Verification items for this drawing (mm, ordinates from the low corner). A direction names the side the tool comes from. Coordinates: 2 decimals unless noted, no trailing zeros. Order: outer loops, then holes, each group sorted by start corner. A loop starts at its lowest first (then second) coordinate and runs counter-clockwise, first axis right, second up. Notation, with made-up numbers: M -7,24 L 6,24 A25 ccw 6,51 Z; hole C 61.5,8.25 d2. An arc over 180 degrees is marked long. One line per item, written item: value. Start each with the question number.
1) Thickness scan on L1, parallel to X at y = 4.05, z = 8; L2, parallel to X at y = 5.75, z = 39; L3, parallel to Z at x = 12, y = 4.25 (1 decimal). Record the ranges inside material, lowest first. Write a range as from..to.
2) Sectioned sample at C-C, the plane x = 3. Enter the section's corners in (y, z) (1 decimal), then the cut area to 3 significant figures.
3) Sectioned sample at B-B, the plane y = 5.25. Enter the section's corners in (x, z) (1 decimal).
4) Sectioned sample at A-A, the plane z = 28. Enter the section's corners in (x, y).
5) Sectioned sample at D-D, the plane x = 33. Enter the section's corners in (y, z) (1 decimal).
6) Go/stop test with flat-tipped pins: P1, Ø16.5, axis at x = 5.5, z = 12, coming from the -Y side; P2, Ø12, axis at x = 5.5, z = 14.5, coming from the +Y side; P3, Ø4, axis at x = 33, y = 1.5, coming from the -Z side (1 decimal). Record where each tip stops, or that it passes through.
7) Access from +Z, -Z, +X, -X, +Y, -Y to the whole of each face (thin tool, end or side, straight path). Record for the marked faces 1, 2 and 3.
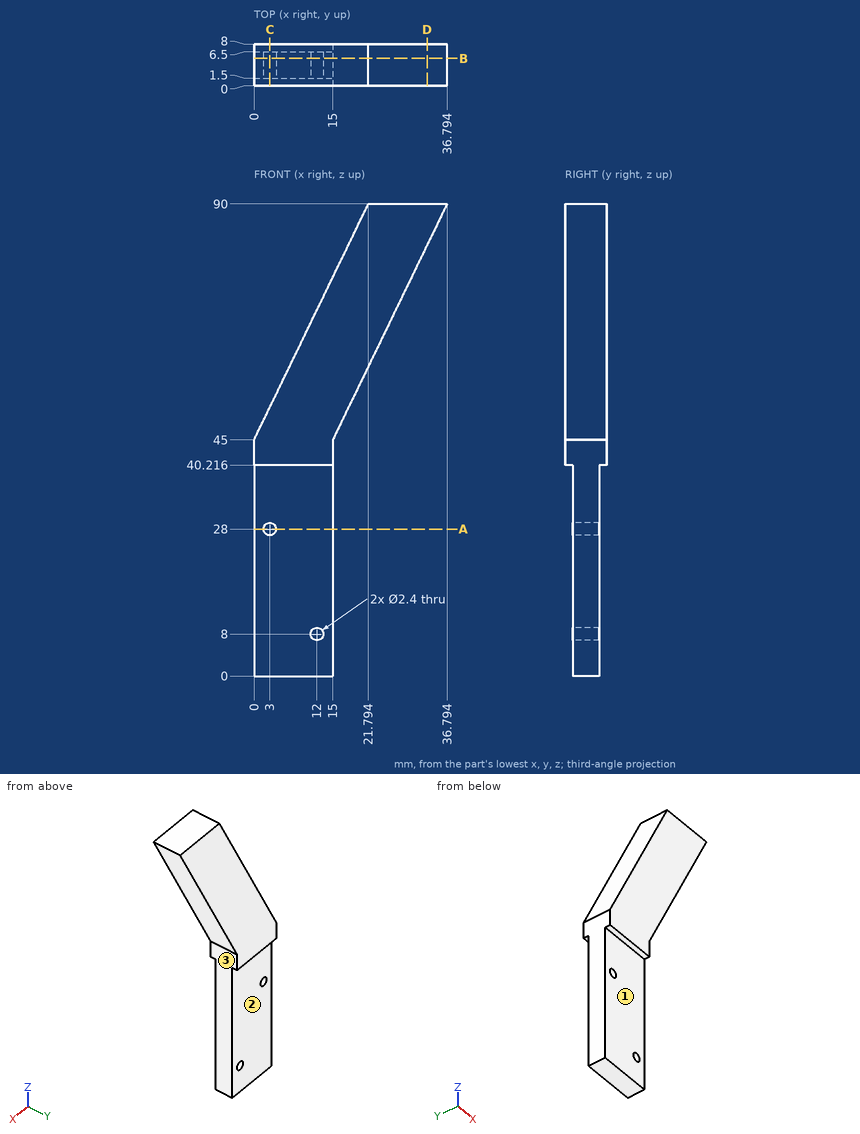
Final values:
1. L1: x = 0..10.8, 13.2..15
1. L2: x = 0..15
1. L3: z = 0..6.8, 9.2..69.8
2. outline: M 0,40.2 L 1.5,40.2 L 1.5,29.2 L 6.5,29.2 L 6.5,40.2 L 8,40.2 L 8,51.2 L 0,51.2 Z; M 1.5,0 L 6.5,0 L 6.5,26.8 L 1.5,26.8 Z
2. area: 277 mm^2
3. outline: M 0,0 L 15,0 L 15,45 L 36.8,90 L 21.8,90 L 0,45 Z; hole C 3,28 d2.4; hole C 12,8 d2.4
4. outline: M 0,1.5 L 1.8,1.5 L 1.8,6.5 L 0,6.5 Z; M 4.2,1.5 L 15,1.5 L 15,6.5 L 4.2,6.5 Z
5. outline: M 0,82.2 L 8,82.2 L 8,90 L 0,90 Z
6. P1: stops at y = 1.5
6. P2: stops at y = 6.5
6. P3: stops at z = 78
7. face 1: -Z, +X, -X, -Y
7. face 2: -Z, +X, -X, +Y
7. face 3: -Z, +X, +Y, -Y
